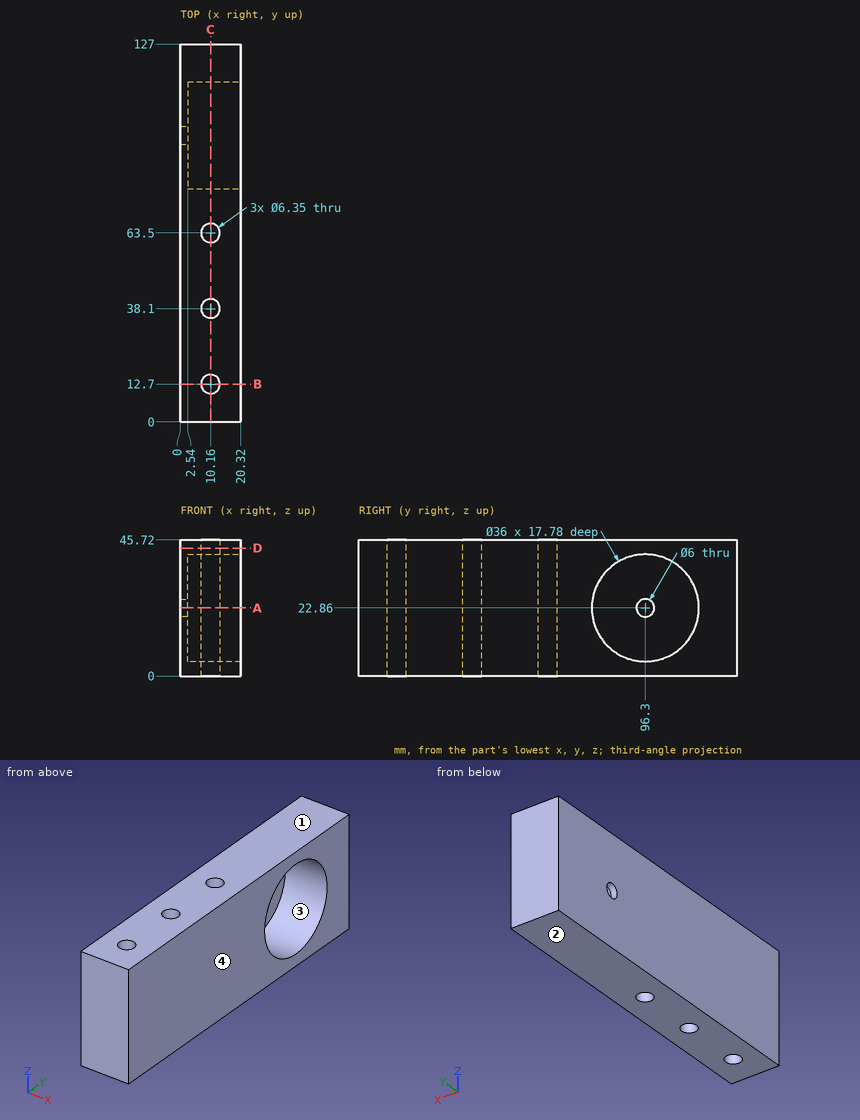
Part print with two shaded views. Sizes in mm from the minimum x, y, z corner. Round coordinates to 2 decimals unless told otherwise and drop trailing zeros. Loops run counter-clockwise (first coordinate to the right, second up) from the corner with the lowest first, then second, coordinate; pieces in that order, holes last.
Item 1: Two-plate mould, pull along Z, no slides. Class the marked faces 1, 2, 3 and 4: released by +Z, released by -Z, zero draft, split by the parting line, or undercut.
Item 2: Pin check, flat tips, straight feed: P1, Ø5, axis at x = 10.16, y = 38.1, coming from the -Z side (1 decimal); P2, Ø9.5, axis at y = 96.3, z = 22.86, coming from the +X side. Stop position of each tip, or through.
Item 3: Saw through at D-D (z = 43). List the corners of the cut face in (x, y) (3 decimals), then the cut area to 3 significant figures.
Item 4: Drill centre lines: line 1 along Y through (x, z) = (12, 32); line 2 along Y through (x, z) = (10.75, 9.5); line 3 along Y through (x, z) = (0.65, 22.86). Where is each one in solid material? Low to high.
Item 5: Saw through at B-B (y = 12.7). List the corners of the cut face in (x, z) (3 decimals), then the cut area to 3 significant figures.
Item 6: Saw through at A-A (z = 22.86). List the corners of the cut face in (x, y) (3 decimals).
Item 7: Saw through at C-C (x = 10.16). List the corners of the cut face in (y, z) (3 decimals).
Worked answers:
1. face 1: released by +Z
1. face 2: released by -Z
1. face 3: undercut
1. face 4: zero draft
2. P1: passes through
2. P2: stops at x = 2.54
3. outline: (0, 0) - (20.32, 0) - (20.32, 127) - (0, 127) - close; hole circle Ø6.35 at (10.16, 12.7); hole circle Ø6.35 at (10.16, 38.1); hole circle Ø6.35 at (10.16, 63.5)
3. area: 2,490 mm2
4. line 1: y = 0 to 10.11, 15.29 to 35.51, 40.69 to 60.91, 66.09 to 80.79, 111.81 to 127
4. line 2: y = 0 to 9.58, 15.82 to 34.98, 41.22 to 60.38, 66.62 to 84.24, 108.36 to 127
4. line 3: y = 0 to 93.3, 99.3 to 127
5. outline: (0, 0) - (6.985, 0) - (6.985, 45.72) - (0, 45.72) - close; (13.335, 0) - (20.32, 0) - (20.32, 45.72) - (13.335, 45.72) - close
5. area: 639 mm2
6. outline: (0, 0) - (20.32, 0) - (20.32, 78.3) - (2.54, 78.3) - (2.54, 93.3) - (0, 93.3) - close; (0, 99.3) - (2.54, 99.3) - (2.54, 114.3) - (20.32, 114.3) - (20.32, 127) - (0, 127) - close; hole circle Ø6.35 at (10.16, 12.7); hole circle Ø6.35 at (10.16, 38.1); hole circle Ø6.35 at (10.16, 63.5)
7. outline: (0, 0) - (9.525, 0) - (9.525, 45.72) - (0, 45.72) - close; (15.875, 0) - (34.925, 0) - (34.925, 45.72) - (15.875, 45.72) - close; (41.275, 0) - (60.325, 0) - (60.325, 45.72) - (41.275, 45.72) - close; (66.675, 0) - (127, 0) - (127, 45.72) - (66.675, 45.72) - close; hole circle Ø36 at (96.3, 22.86)
